Study the drawing (mm; zero at the part's minimum x, y, z) and answer. A direction names the side the tool comes from. Coordinates: 2 decimals unless noted, no trailing zeros. Write each loop counter-clockwise with the first axis right and the second up, starting at its lowest first coordinate (ties: lowest second). Pieces come first, ordered by that corner, then holes. Notation, with made-up numbers: (-33.5, -26) -> (11.5, -26) arc R10 cw to (11.5, -18) -> close; hole circle Ø3 at (-2, -30). An arc over 180 degrees is marked (long way). Write each question's results on one line, items separated by ' | '. Start each with the question number.
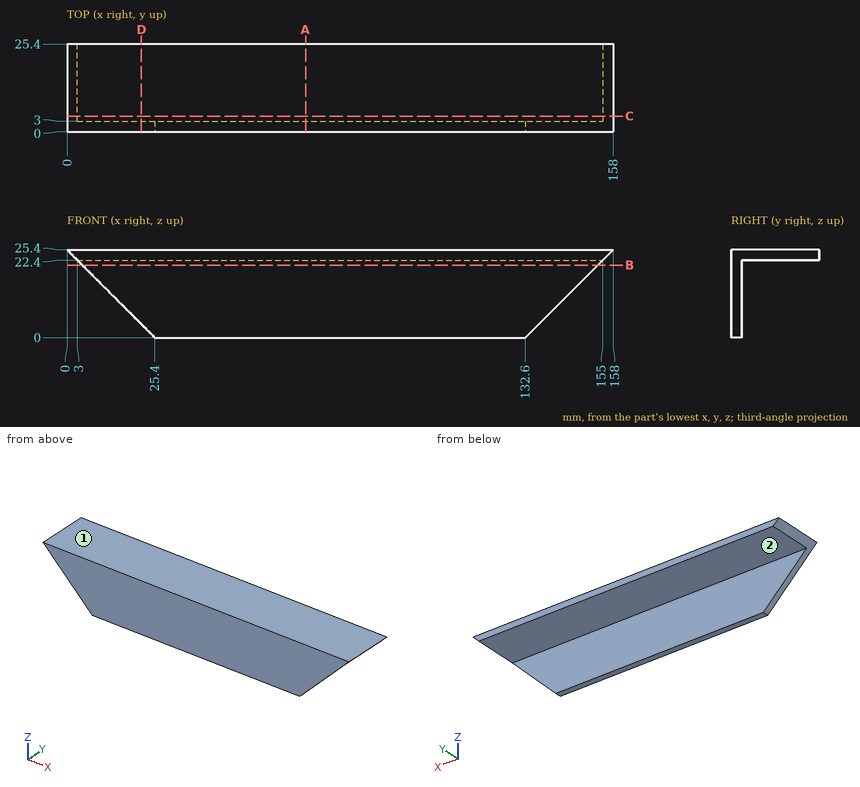
1. For the marked faces 1 and 2, determine the directions among +Z, -Z, +X, -X, +Y, -Y from which every point of the face is accessible in a straight line to the end or side of a thin tool.
2. Find section D-D on x = 21.5. Give the vertices of the cut face in (y, z).
3. Given pin 1 Ø1 at (x, z) = (89, 5.5) entering from +Y; pin 2 Ø11 at (x, y) = (86.5, 13.5) entering from -Z; pin 3 Ø3 at (y, z) = (3, 10) entering from -X, each flat-ended and moving along its own axis, determine where each tip first touches the part or whether it passes through.
4. Find section A-A on x = 69. Give the vertices of the cut face in (y, z), and give its area (3 significant figures).
5. Find the intervals of material crossed by L1, parallel to Z at x = 48, y = 12.25; L2, parallel to Y at x = 89, z = 1.5, in increasing order.
6. Find section B-B on z = 21. Give the vertices of the cut face in (x, y).
7. Find section C-C on y = 4.5. Give the vertices of the cut face in (x, z).
Ans:
1) face 1: +Z, +X, -X, +Y, -Y | face 2: -Z, +X, -X, +Y
2) outline: (0, 3.9) -> (3, 3.9) -> (3, 22.4) -> (25.4, 22.4) -> (25.4, 25.4) -> (0, 25.4) -> close
3) pin 1: stops at y = 3 | pin 2: stops at z = 22.4 | pin 3: stops at x = 13.9
4) outline: (0, 0) -> (3, 0) -> (3, 22.4) -> (25.4, 22.4) -> (25.4, 25.4) -> (0, 25.4) -> close | area: 143 mm²
5) L1: z = 22.4 to 25.4 | L2: y = 0 to 3
6) outline: (4.4, 0) -> (153.6, 0) -> (153.6, 3) -> (4.4, 3) -> close
7) outline: (0, 25.4) -> (3, 22.4) -> (155, 22.4) -> (158, 25.4) -> close
